from build123d import *

# Parameters (mm, degrees)
EXTRUDE_1_DEPTH      = 5.8
SKETCH_2_W           = 9
SKETCH_2_H           = 4.8
CUT_EXTRUDE_1_DEPTH  = 6
SKETCH_3_W           = 0.6
SKETCH_3_H           = 0.6
EXTRUDE_2_DEPTH      = 2.4
EXTRUDE_2_DEPTH_BACK = 6.1
SKETCH_5_W           = 7
SKETCH_5_H           = 4
CUT_EXTRUDE_2_DEPTH  = 1
SKETCH_6_W           = 0.6
SKETCH_6_H           = 0.6
EXTRUDE_3_DEPTH      = 6


with BuildPart() as part:
    # 草图1 → 凸台-拉伸1 (new body)
    with BuildSketch(Plane.XY):
        Polygon((2.75, 0), (2.75, 0.5), (4.75, 0.5), (4.75, 0), (5.25, 0), (5.25, 0.5), (7.25, 0.5), (7.25, 0), (10, 0), (10, 7), (0, 7), (0, 0), align=None)
    extrude(amount=EXTRUDE_1_DEPTH)

    # 草图2 → 切除-拉伸1 (cut)
    with BuildSketch(Plane(origin=(0, 7, 0), x_dir=(1, 0, 0), z_dir=(0, 1, 0))):
        with Locations((5, -2.9)):
            Rectangle(SKETCH_2_W, SKETCH_2_H)
    extrude(amount=-CUT_EXTRUDE_1_DEPTH, mode=Mode.SUBTRACT)

    # 草图3 → 凸台-拉伸2 (add, two sides)
    with BuildSketch(Plane.XZ) as extrude_2_sk:
        with Locations((2.46, 3.4)):
            Rectangle(SKETCH_3_W, SKETCH_3_H)
        with Locations((5, 3.4)):
            Rectangle(SKETCH_3_W, SKETCH_3_H)
        with Locations((7.54, 3.4)):
            Rectangle(SKETCH_3_W, SKETCH_3_H)
    extrude(amount=EXTRUDE_2_DEPTH)
    extrude(extrude_2_sk.sketch, amount=-EXTRUDE_2_DEPTH_BACK)

    # 草图5 → 切除-拉伸2 (cut)
    with BuildSketch(Plane.XY.offset(5.8)):
        with Locations((5, 5)):
            Rectangle(SKETCH_5_W, SKETCH_5_H)
    extrude(amount=-CUT_EXTRUDE_2_DEPTH, mode=Mode.SUBTRACT)

    # 草图6 → 凸台-拉伸3 (add)
    with BuildSketch(Plane(origin=(0, 0, 3.1), x_dir=(-1, 0, 0), z_dir=(0, 0, -1))):
        with Locations((-2.46, -2.1)):
            Rectangle(SKETCH_6_W, SKETCH_6_H)
        with Locations((-5, -2.1)):
            Rectangle(SKETCH_6_W, SKETCH_6_H)
        with Locations((-7.54, -2.1)):
            Rectangle(SKETCH_6_W, SKETCH_6_H)
    extrude(amount=EXTRUDE_3_DEPTH)


solid = part.part
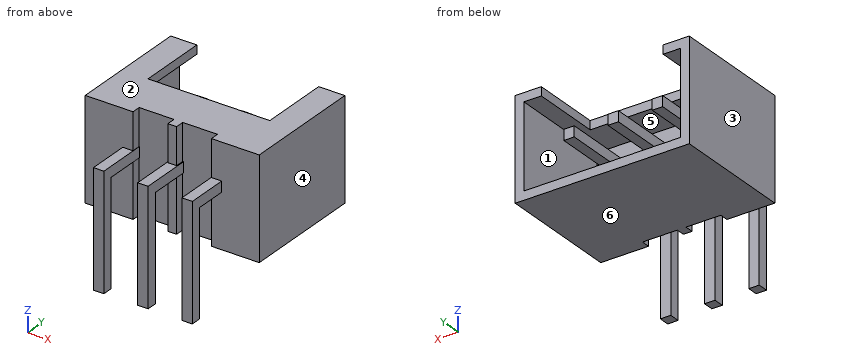
Design review of the part built by this model. Coordinates are the model's own, in mm. Face numbers are marked on the shaded views. A direction names the side the tool comes from. Give positions to 0.01 mm unless a question says otherwise; leave off trailing zeros. Write each loop counter-clockwise with the first axis right and the second up, starting at its lowest first coordinate (ties: lowest second). Pieces come first, ordered by that corner, then holes. Notation, with made-up numbers: M 39.5,32 L 71.5,32 A22 cw 71.5,53 Z; hole C -32.75,-12 d2. An arc over 180 degrees is marked long. Return JSON: item names as keys, results as strings. Group by question number.
Item 1: Take a section at C-C (z = 0.25). Give the boundary of the cut face in (x, y), plus the area to 3 significant figures.
Item 2: Take a section at D-D (x = 3.5). Give the boundary of the cut face in (y, z).
Item 3: Tool access review of the marked faces 1 and 2: name each direction out of +Z, -Z, +X, -X, +Y, -Y from which nothing blocks a thin tool from reaching the whole face with its end or side.
Item 4: Take a section at B-B (y = 0.25). Count the separate pieces of the cut face and the enclosed holes in it, plus the area to 3 significant figures.
Item 5: Take a section at A-A (z = -1.25). Give the boundary of the cut face in (x, y).
Item 6: Wall thickness on line 1 along X through (y, z) = (0.25, 2.25); line 2 along Z through (x, y) = (2.25, 2.5); line 3 along Z through (x, y) = (2.5, 5.25): over which ranges is each line inside the solid? List them lowest first.
Item 7: The part is to be moulded in two halves that separate along X. For the marked faces 3, 4, 5 and 6, say which applies: pulls with the +X half, pulls with the -X half, needs draft (parallel to the pull), parting line crosses it, or undercut.
Item 8: Clearance check with flat-ended pins moving along their axes: pin 1 Ø1.5 at (y, z) = (3, -1) entering from +X; pin 2 Ø2.5 at (y, z) = (-1.5, 1.5) entering from +X; pin 3 Ø0.5 at (x, y) = (2.5, 3.5) entering from +Z. State where each tip first meets the part, or that it passes through.
Return value:
{
 "1": {"outline": "M 0,0 L 2.75,0 L 2.75,0.5 L 4.75,0.5 L 4.75,0 L 5.25,0 L 5.25,0.5 L 7.25,0.5 L 7.25,0 L 10,0 L 10,7 L 0,7 Z; M 2.16,-2.4 L 2.76,-2.4 L 2.76,-1.8 L 2.16,-1.8 Z; M 4.7,-2.4 L 5.3,-2.4 L 5.3,-1.8 L 4.7,-1.8 Z; M 7.24,-2.4 L 7.84,-2.4 L 7.84,-1.8 L 7.24,-1.8 Z", "area": "69.1 mm2"},
 "2": {"outline": "M 0.5,0 L 7,0 L 7,0.5 L 1,0.5 L 1,5.3 L 3,5.3 L 3,5.8 L 0.5,5.8 Z"},
 "3": {"face 1": "+Y", "face 2": "+Z, +X, -X, +Y, -Y"},
 "4": {"separate pieces": "3", "enclosed holes": "0", "area": "34.9 mm2"},
 "5": {"outline": "M 2.16,-2.4 L 2.76,-2.4 L 2.76,-1.8 L 2.16,-1.8 Z; M 4.7,-2.4 L 5.3,-2.4 L 5.3,-1.8 L 4.7,-1.8 Z; M 7.24,-2.4 L 7.84,-2.4 L 7.84,-1.8 L 7.24,-1.8 Z"},
 "6": {"line 1": "x = 0 to 2.75, 4.75 to 5.25, 7.25 to 10", "line 2": "z = 0 to 0.5, 3.1 to 3.7, 5.3 to 5.8", "line 3": "z = 0 to 0.5, 3.1 to 3.7"},
 "7": {"face 3": "pulls with the -X half", "face 4": "pulls with the +X half", "face 5": "undercut", "face 6": "needs draft"},
 "8": {"pin 1": "passes through", "pin 2": "stops at x = 7.84", "pin 3": "stops at z = 3.7"}
}
